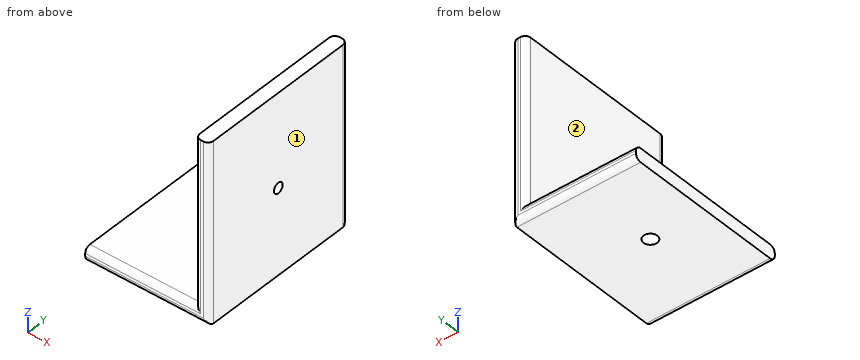
```python
from build123d import *

# Parameters (mm, degrees)
F1_DEPTH = 152.4
F3_D     = 9.525
F5_D     = 12.7
F6_R     = 5.08
F7_R     = 5.08
F8_R     = 5.08
F9_R     = 5.08


# Not quite as in the source:
# - a length typed as a fraction of an inch, garbled in the dataset ("3 / 203.2 mm" for 3/8 in), is restored


with BuildPart() as f1:
    # F0 (on Front) → F1 (new body)
    with BuildSketch(Plane.XZ):
        Polygon((0, -78.9952108244), (0, 86.1047891756), (-12.7, 86.1047891756), (-12.7, -66.2952108244), (-114.3, -66.2952108244), (-114.3, -78.9952108244), align=None)
    extrude(amount=F1_DEPTH)

    # F3 (through all)
    with Locations(Plane.YZ):
        with Locations((-76.2, 0)):
            Hole(F3_D / 2)

    # F5 (through all)
    with Locations(Plane.XY.offset(-66.2952108244)):
        with Locations((-63.5, -76.2)):
            Hole(F5_D / 2)

    # F6
    f6_edges = [f1.edges().sort_by_distance(p)[0] for p in [
        (-12.7, -152.4, 9.904789),
        (-63.5, -152.4, -66.295211),
    ]]
    fillet(f6_edges, radius=F6_R)

    # F7
    f7_edges = [f1.edges().sort_by_distance(p)[0] for p in [
        (-12.7, 0, 9.904789),
        (-63.5, 0, -66.295211),
    ]]
    fillet(f7_edges, radius=F7_R)

    # F8
    f8_edges = [f1.edges().sort_by_distance(p)[0] for p in [
        (-57.15, 0, -78.995211),
        (0, 0, 3.554789),
    ]]
    fillet(f8_edges, radius=F8_R)

    # F9
    f9_edges = [f1.edges().sort_by_distance(p)[0] for p in [
        (-57.15, -152.4, -78.995211),
        (0, -152.4, 3.554789),
    ]]
    fillet(f9_edges, radius=F9_R)


solid = f1.part
```
Work out the finished part from the listing and answer in its coordinate system (mm). Face numbers are marked on the shaded views. A direction names the side the tool comes from. Give positions to 0.01 mm unless a question says otherwise; leave off trailing zeros. Loops run counter-clockwise (first coordinate to the right, second up) from the corner with the lowest first, then second, coordinate; pieces in that order, holes last. Notation, with made-up numbers: (38.25, 43) -> (97.25, 43) arc R20 cw to (97.25, 71) -> close; hole circle Ø6 at (88.25, -36.5). An arc over 180 degrees is marked (long way). One line per question, with ' | ' between items. Start each with the question number.
1) Straight lines are drawn through the part: L1, parallel to Z at x = -4.5, y = -76.2; L2, parallel to Y at x = -63.5, z = -72.25; L3, parallel to Z at x = -82.5, y = -78. For each, find the intervals that lie inside material, in ascending order.
2) Section B-B, the plane x = -63.5 is taken. Determine the outline of the cut face in (y, z).
3) Section A-A, the plane z = 0 is taken. Determine the outline of the cut face in (x, y), then the cut area to 3 significant figures.
4) Each of these flat-tipped pins is pushed along its axis until it touches: pin 1 (1 mm diameter, centred on y = -115, z = 39.5, fed in from -X); pin 2 (16.5 mm diameter, centred on x = -63.5, y = -76.2, fed in from +Z). Where does it stop, or does it pass through?
5) For the marked faces 1 and 2, determine the directions among +Z, -Z, +X, -X, +Y, -Y from which every point of the face is accessible in a straight line to the end or side of a thin tool.
6) Section D-D, the plane z = 59 is taken. Determine the outline of the cut face in (x, y), then the cut area to 3 significant figures.
7) Section C-C, the plane y = -76.2 is taken. Determine the outline of the cut face in (x, z), then the cut area to 3 significant figures.
Resolved:
1) L1: -79 to -4.76, 4.76 to 86.1 | L2: -152.4 to -82.55, -69.85 to 0 | L3: -79 to -66.3
2) outline: (-152.4, -73.92) arc R5.08 ccw to (-147.32, -79) -> (-82.55, -79) -> (-82.55, -66.3) -> (-147.32, -66.3) arc R5.08 ccw to (-152.4, -71.38) -> close; (-69.85, -79) -> (-5.08, -79) arc R5.08 ccw to (0, -73.92) -> (0, -71.38) arc R5.08 ccw to (-5.08, -66.3) -> (-69.85, -66.3) -> close
3) outline: (-12.7, -147.32) arc R5.08 ccw to (-7.62, -152.4) -> (-5.08, -152.4) arc R5.08 ccw to (0, -147.32) -> (0, -80.96) -> (-12.7, -80.96) -> close; (-12.7, -71.44) -> (0, -71.44) -> (0, -5.08) arc R5.08 ccw to (-5.08, 0) -> (-7.62, 0) arc R5.08 ccw to (-12.7, -5.08) -> close | area: 1,790 mm2
4) pin 1: x = -12.7 | pin 2: z = -66.3
5) face 1: +Z, -Z, +X, +Y, -Y | face 2: +Z, -X, +Y, -Y
6) outline: (-12.7, -147.32) arc R5.08 ccw to (-7.62, -152.4) -> (-5.08, -152.4) arc R5.08 ccw to (0, -147.32) -> (0, -5.08) arc R5.08 ccw to (-5.08, 0) -> (-7.62, 0) arc R5.08 ccw to (-12.7, -5.08) -> close | area: 1,910 mm2
7) outline: (-114.3, -79) -> (-69.85, -79) -> (-69.85, -66.3) -> (-114.3, -66.3) -> close; (-57.15, -79) -> (0, -79) -> (0, -4.76) -> (-12.7, -4.76) -> (-12.7, -66.3) -> (-57.15, -66.3) -> close; (-12.7, 4.76) -> (0, 4.76) -> (0, 86.1) -> (-12.7, 86.1) -> close | area: 3,100 mm2
